Geometry check sheet. Reference: drawing and pictorial views, mm from the part's lowest x, y, z. Round coordinates to 2 decimals unless told otherwise and drop trailing zeros. Write each loop counter-clockwise with the first axis right and the second up, starting at its lowest first coordinate (ties: lowest second). Pieces come first, ordered by that corner, then holes. Notation, with made-up numbers: M -21.75,76.5 L 24.25,76.5 A23 ccw 24.25,105.5 Z; hole C 58.5,23 d9. An arc over 180 degrees is marked long. Use a Markdown table: item, result. Add a question column.
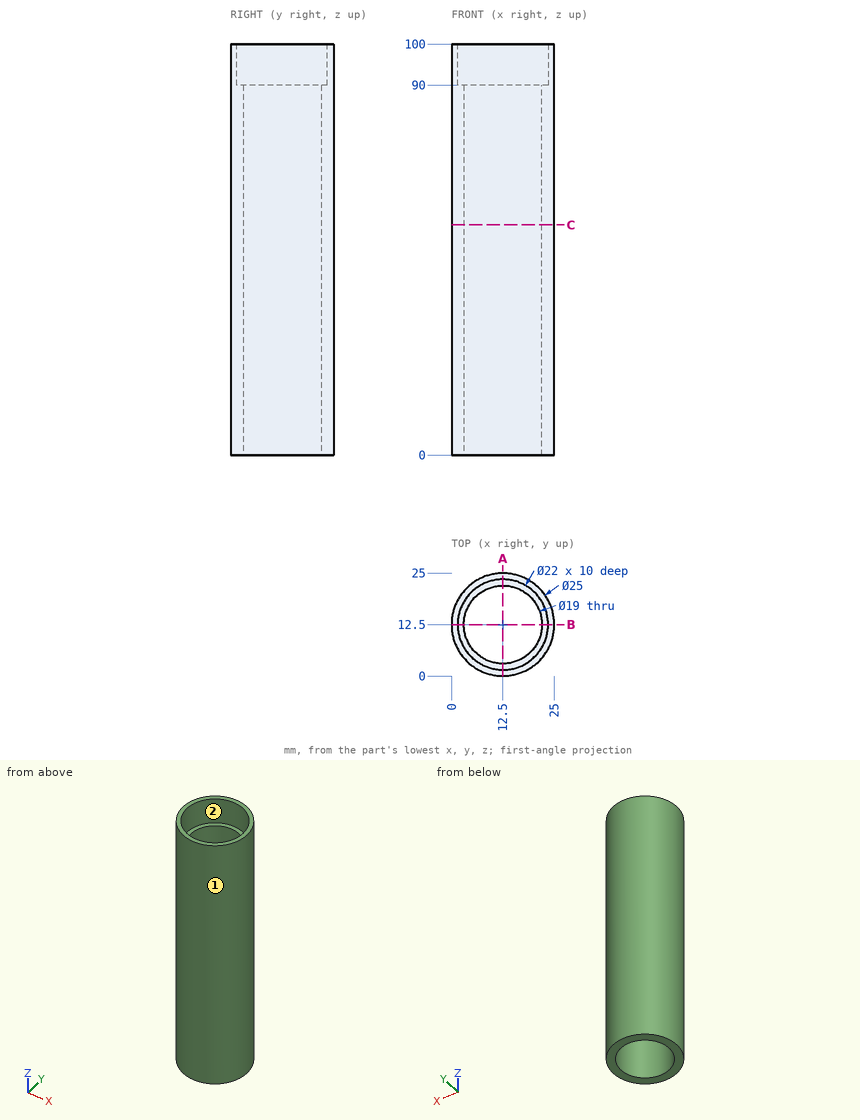
1. Cross-section at A-A on x = 12.5. Enter the section's corners in (y, z), plus the area to 3 significant figures.
2. Depth check by flat-ended pin: pin 1 Ø2 at (y, z) = (21, 78.5) entering from +X; pin 2 Ø3 at (y, z) = (14.5, 84) entering from +X; pin 3 Ø1.5 at (x, z) = (21.5, 69) entering from -Y; pin 4 Ø12 at (x, y) = (12.5, 4.5) entering from +Z. Enter the tip coordinate at first touch or a pass-through.
3. Release check for a two-part mould opening along X. For the marked faces 1 and 2 record: +X half, -X half, draft (parallel to the pull), parting line (faces both ways), or undercut.
4. Cross-section at C-C on z = 56. Enter the section's corners in (x, y), plus the area to 3 significant figures.
5. Scan lines: line 1 along Y through (x, z) = (12.5, 26.5); line 2 along Z through (x, y) = (20.75, 6.5). Record each from-to range of solid material in increasing order. Write a range as from..to.
Answer:
| question | item | result |
|---|---|---|
| 1 | outline | M 0,0 L 3,0 L 3,90 L 1.5,90 L 1.5,100 L 0,100 Z; M 22,0 L 25,0 L 25,100 L 23.5,100 L 23.5,90 L 22,90 Z |
| 1 | area | 570 mm^2 |
| 2 | pin 1 | stops at x = 22.5 |
| 2 | pin 2 | stops at x = 24.99 |
| 2 | pin 3 | stops at y = 3.11 |
| 2 | pin 4 | stops at z = 100 |
| 3 | face 1 | parting line |
| 3 | face 2 | undercut |
| 4 | outline | C 12.5,12.5 d25; hole C 12.5,12.5 d19 |
| 4 | area | 207 mm^2 |
| 5 | line 1 | y = 0..3, 22..25 |
| 5 | line 2 | z = 0..90 |
